Can you work these out from the model? Positions are in its coordinate system, mm. A direction names the side the tool comes from. Coordinates: 2 decimals unless noted, no trailing zeros. Loops run counter-clockwise (first coordinate to the right, second up) from the corner with the lowest first, then second, coordinate; pieces in that order, holes last. Notation, with made-up numbers: M 58.25,-28.5 L 115.25,-28.5 A24 ccw 115.25,-0.5 Z; hole C 48,62.25 d1. An arc over 180 degrees is marked long. Answer as a JSON object with one key per item and string values. Group by question number.
Item 1: Which directions (+Z, -Z, +X, -X, +Y, -Y) give clear straight access to the entire face, cutting with the end or side of a thin tool? Please do faces 5 (the cylindrical face through (1.29, 7.465, 2.024)), 6 (the flat face through (2.028, -0.07, 3.448)).
Item 2: Suppose I cut it at C-C (z = 0). Write out the boundary of the cut face in (x, y), then the cut area to 3 significant figures.
Item 3: Suppose I cut it at B-B (x = 1). Write out the boundary of the cut face in (y, z), then the cut area to 3 significant figures.
Item 4: Suppose I cut it at A-A (y = -3). Write out the boundary of the cut face in (x, z).
Item 5: I'm going to push a flat-ended pin straight in: pin 1 Ø3 at (x, z) = (0, 0) entering from +Y. Where does the tip first touch, or does it pass through?
Item 6: Suppose I cut it at D-D (y = 8). Write out the boundary of the cut face in (x, z).
Item 7: We'd pull the mould along X, two halves only. Please class faces 1 (the flat face through (1.97, -0.07, -3.48)), 2 (the cylindrical face through (-0.125, 2.395, -1.896)), 3 (the flat face through (-4, 0, 0)), 4 (the flat face through (-2, 5, -2)): +X half, -X half, draft (parallel to the pull), parting line (faces both ways), or undercut.
Item 8: If I drill on line 1 (X direction, y = -1.5, z = 0); line 2 (Y direction, x = 1.25, z = -3); line 3 (Z direction, x = 1.5, y = 9), over which ranges is the centre line in solid material (lowest first)?
Autodesk Inventor part; units mm, degrees
ref_plane "YZ Plane" through (0, 0, 0) normal (1, 0, 0) x (0, 1, 0)
ref_plane "XZ Plane" through (0, 0, 0) normal (0, 1, 0) x (-1, 0, 0)
ref_plane "XY Plane" through (0, 0, 0) normal (0, 0, 1) x (1, 0, 0)
sketch "Boceto1" plane through (0, 0, 0) normal (0, 1, 0) x (-1, 0, 0)
  line L0 (0, 4.6188) -> (4, 2.3094)
  line L1 (4, 2.3094) -> (4, -2.3094)
  line L2 (4, -2.3094) -> (0, -4.6188)
  line L3 (0, -4.6188) -> (-4, -2.3094)
  line L4 (-4, -2.3094) -> (-4, 2.3094)
  line L5 (-4, 2.3094) -> (0, 4.6188)
  circle A0 centre (0, 0) radius 1.9
  point P0 (4, 0)
  dimension "d0" = 3.8
  dimension "d2" = 4
extrude "Extrusión1" add sketch "Boceto1" along normal mid plane 10
sketch "Boceto2" plane through (0, 5, 0) normal (0, 1, 0) x (1, 0, 0)
  circle A0 centre (0, 0) radius 1.9
  circle A1 centre (0, 0) radius 2.4
  dimension "d5" = 4.8
extrude "Extrusión2" add sketch "Boceto2" along normal blind 5
properties part number "expansor de conexion"
From the geometry:
{
 "1": {"face 5": "+Y", "face 6": "+Z, +X, +Y, -Y"},
 "2": {"outline": "M -4,-5 L -1.9,-5 L -1.9,10 L -2.4,10 L -2.4,5 L -4,5 Z; M 1.9,-5 L 4,-5 L 4,5 L 2.4,5 L 2.4,10 L 1.9,10 Z", "area": "47.0 mm2"},
 "3": {"outline": "M -5,-4.04 L 5,-4.04 L 5,-2.18 L 10,-2.18 L 10,-1.62 L -5,-1.62 Z; M -5,1.62 L 10,1.62 L 10,2.18 L 5,2.18 L 5,4.04 L -5,4.04 Z", "area": "54.2 mm2"},
 "4": {"outline": "M -4,-2.31 L 0,-4.62 L 4,-2.31 L 4,2.31 L 0,4.62 L -4,2.31 Z; hole C 0,0 d3.8"},
 "5": {"pin 1": "through"},
 "6": {"outline": "C 0,0 d4.8; hole C 0,0 d3.8"},
 "7": {"face 1": "+X half", "face 2": "undercut", "face 3": "-X half", "face 4": "draft"},
 "8": {"line 1": "-4 to -1.9, 1.9 to 4", "line 2": "-5 to 5", "line 3": "-1.87 to -1.17, 1.17 to 1.87"}
}
